Verification items for the finished model (mm, model axes). Give positions to 0.01 mm unless a question says otherwise; leave off trailing zeros. Write each loop counter-clockwise with the first axis right and the second up, starting at its lowest first coordinate (ties: lowest second). Pieces come first, ordered by that corner, then holes. Notation, with made-up numbers: (47.25, 21) - (106.25, 21) arc R19 ccw to (106.25, 43) - close; hole circle Ø9 at (11.25, 71). An arc over 180 degrees is marked (long way). Answer as a JSON object with one key per item and string values. Group by question number.
Item 1: Sectioned sample at A-A, the plane x = -47. Record the boundary of the cut face in (y, z).
Item 2: Go/stop test with flat-tipped pins: pin 1 (1.5 mm diameter, centred on y = 5.5, z = 56, fed in from +X); pin 2 (1.5 mm diameter, centred on x = 38.5, y = 4.5, fed in from -Z); pin 3 (4 mm diameter, centred on y = 3.5, z = -37.5, fed in from -X). Record where each tip stops, or that it passes through.
Item 3: Sectioned sample at B-B, the plane z = 57. Record the boundary of the cut face in (x, y).
Item 4: Scan line: line 1 along Z through (x, y) = (43, 6.25). Record every from-to range of solid material in increasing order. Write a range as [from, to].
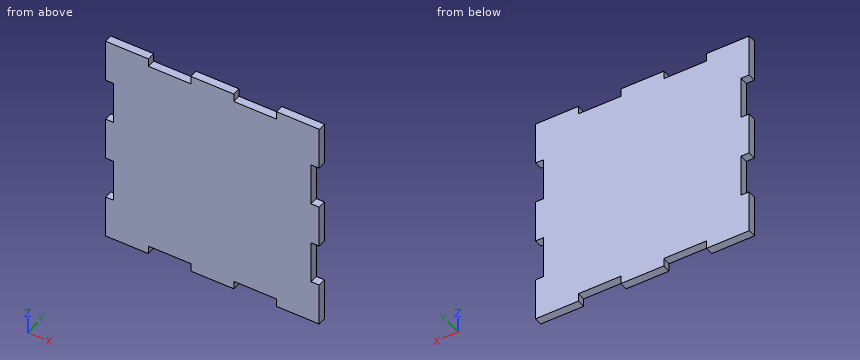
Autodesk Inventor part; units mm, degrees
ref_plane "YZ Plane" through (0, 0, 0) normal (1, 0, 0) x (0, 1, 0)
ref_plane "XZ Plane" through (0, 0, 0) normal (0, 1, 0) x (-1, 0, 0)
ref_plane "XY Plane" through (0, 0, 0) normal (0, 0, 1) x (1, 0, 0)
sketch "Sketch2" plane through (0, 0, 0) normal (0, 1, 0) x (-1, 0, 0)
  line L0 (-105, 105) -> (105, 105)
  line L1 (105, 105) -> (105, -105)
  line L2 (105, -105) -> (-105, -105)
  line L3 (-105, -105) -> (-105, 105)
  line L4 (-105, 105) -> (105, -105) construction
  line L5 (105, 105) -> (-105, -105) construction
  point P0 (0, 0)
  dimension "d11" = 210
  dimension "d12" = 210
extrude "Extrusion2" add sketch "Sketch2" along normal blind 8
sketch "Sketch4" plane through (0, 0, 0) normal (0, -1, 0) x (1, 0, 0)
  line L0 (105, 105) -> (-105, 105)
  line L1 (-105, 105) -> (-105, -105)
  line L2 (-105, -105) -> (105, -105)
  line L3 (105, -105) -> (105, 105)
  line L4 (-105, -63) -> (-97, -63)
  line L5 (-97, -63) -> (-97, -21)
  line L6 (-97, -21) -> (-105, -21)
  line L7 (-105, -21) -> (-105, -63)
  line L8 (-105, 21) -> (-97, 21)
  line L9 (-97, 21) -> (-97, 63)
  line L10 (-97, 63) -> (-105, 63)
  line L11 (-105, 63) -> (-105, 21)
  line L12 (-97, -21) -> (-97, 21) construction
  line L13 (-97, 63) -> (-97, 105) construction
  line L14 (-97, -63) -> (-97, -105)
  point P0 (0, 0)
  dimension "d27" = 8
extrude "Extrusion3" cut sketch "Sketch4" against normal through all contours L10 L9 L8 L1 | L4 L1 L6 L5
sketch "Sketch5" plane through (0, 0, 0) normal (0, -1, 0) x (1, 0, 0)
  line L0 (-97, 21) -> (-105, 21)
  line L1 (-105, 21) -> (-105, -21)
  line L2 (-105, -21) -> (-97, -21)
  line L3 (-97, -21) -> (-97, -63)
  line L4 (-97, -63) -> (-105, -63)
  line L5 (-105, -63) -> (-105, -105)
  line L6 (-105, -105) -> (105, -105)
  line L7 (105, -105) -> (105, 105)
  line L8 (105, 105) -> (-105, 105)
  line L9 (-105, 105) -> (-105, 63)
  line L10 (-105, 63) -> (-97, 63)
  line L11 (-97, 63) -> (-97, 21)
  line L12 (63, -105) -> (21, -105)
  line L13 (21, -105) -> (21, -97)
  line L14 (21, -97) -> (63, -97)
  line L15 (63, -97) -> (63, -105)
  line L16 (-21, -105) -> (-63, -105)
  line L17 (-63, -105) -> (-63, -97)
  line L18 (-63, -97) -> (-21, -97)
  line L19 (-21, -97) -> (-21, -105)
  line L20 (63, -97) -> (105, -97) construction
  line L21 (21, -97) -> (-21, -97) construction
  line L22 (-63, -97) -> (-105, -97) construction
  point P0 (0, 0)
  dimension "d31" = 8
extrude "Extrusion4" cut sketch "Sketch5" against normal through all contours L6 L13 L14 L15 | L17 L18 L19 L6
mirror "Mirror1" about plane through (0, 0, 0) normal (1, 0, 0) of "Extrusion3"
mirror "Mirror2" about plane through (0, 0, 0) normal (0, 0, 1) of "Extrusion4"
equation "\"d11\" = d12"
properties part number "M01 - Base Top" material "Wood (Walnut)"
Geometry check:
{
 "1": {"outline": "(0, -97) - (8, -97) - (8, 97) - (0, 97) - close"},
 "2": {"pin 1": "x = 97", "pin 2": "z = -97", "pin 3": "x = -97"},
 "3": {"outline": "(-97, 0) - (97, 0) - (97, 8) - (-97, 8) - close"},
 "4": {"line 1": "[-97, 97]"}
}
